```python
from build123d import *

# Parameters (mm, degrees)
SKETCH1_R           = 2.35
BOSS_EXTRUDE1_DEPTH = 7.8
SKETCH2_R           = 2.7
CUT_EXTRUDE1_DEPTH  = 0.7
SKETCH3_R           = 2.705
CUT_EXTRUDE2_DEPTH  = 0.7


with BuildPart() as part:
    # Sketch1 → Boss-Extrude1 (new body)
    with BuildSketch(Plane(origin=(0, 0, 0), x_dir=(0, 0, -1), z_dir=(1, 0, 0))):
        with BuildLine():
            Line((-48, -3.73), (48, -3.73))
            ThreePointArc((48, -3.73), (51.73, 0), (48, 3.73))
            Line((48, 3.73), (-48, 3.73))
            ThreePointArc((-48, 3.73), (-51.73, 0), (-48, -3.73))
        make_face()
        with Locations((-48, 0)):
            Circle(SKETCH1_R, mode=Mode.SUBTRACT)
        with Locations((-40, 0)):
            Circle(SKETCH1_R, mode=Mode.SUBTRACT)
        with Locations((-32, 0)):
            Circle(SKETCH1_R, mode=Mode.SUBTRACT)
        with Locations((-24, 0)):
            Circle(SKETCH1_R, mode=Mode.SUBTRACT)
        with Locations((-16, 0)):
            Circle(SKETCH1_R, mode=Mode.SUBTRACT)
        with Locations((-8, 0)):
            Circle(SKETCH1_R, mode=Mode.SUBTRACT)
        Circle(SKETCH1_R, mode=Mode.SUBTRACT)
        with Locations((8, 0)):
            Circle(SKETCH1_R, mode=Mode.SUBTRACT)
        with Locations((16, 0)):
            Circle(SKETCH1_R, mode=Mode.SUBTRACT)
        with Locations((24, 0)):
            Circle(SKETCH1_R, mode=Mode.SUBTRACT)
        with Locations((32, 0)):
            Circle(SKETCH1_R, mode=Mode.SUBTRACT)
        with Locations((40, 0)):
            Circle(SKETCH1_R, mode=Mode.SUBTRACT)
        with Locations((48, 0)):
            Circle(SKETCH1_R, mode=Mode.SUBTRACT)
    extrude(amount=BOSS_EXTRUDE1_DEPTH)

    # Sketch2 → Cut-Extrude1 (cut)
    with BuildSketch(Plane(origin=(7.8, 0, 0), x_dir=(0, 0, -1), z_dir=(1, 0, 0))):
        with Locations((-48, 0)):
            Circle(SKETCH2_R)
        with Locations((-40, 0)):
            Circle(SKETCH2_R)
        with Locations((-32, 0)):
            Circle(SKETCH2_R)
        with Locations((-24, 0)):
            Circle(SKETCH2_R)
        with Locations((-16, 0)):
            Circle(SKETCH2_R)
        with Locations((-8, 0)):
            Circle(SKETCH2_R)
        Circle(SKETCH2_R)
        with Locations((8, 0)):
            Circle(SKETCH2_R)
        with Locations((16, 0)):
            Circle(SKETCH2_R)
        with Locations((24, 0)):
            Circle(SKETCH2_R)
        with Locations((32, 0)):
            Circle(SKETCH2_R)
        with Locations((40, 0)):
            Circle(SKETCH2_R)
        with Locations((48, 0)):
            Circle(SKETCH2_R)
    extrude(amount=-CUT_EXTRUDE1_DEPTH, mode=Mode.SUBTRACT)

    # Sketch3 → Cut-Extrude2 (cut)
    with BuildSketch(Plane.ZY):
        with Locations((-48, 0)):
            Circle(SKETCH3_R)
        with Locations((-40, 0)):
            Circle(SKETCH3_R)
        with Locations((-32, 0)):
            Circle(SKETCH3_R)
        with Locations((-24, 0)):
            Circle(SKETCH3_R)
        with Locations((-16, 0)):
            Circle(SKETCH3_R)
        with Locations((-8, 0)):
            Circle(SKETCH3_R)
        Circle(SKETCH3_R)
        with Locations((8, 0)):
            Circle(SKETCH3_R)
        with Locations((16, 0)):
            Circle(SKETCH3_R)
        with Locations((24, 0)):
            Circle(SKETCH3_R)
        with Locations((32, 0)):
            Circle(SKETCH3_R)
        with Locations((40, 0)):
            Circle(SKETCH3_R)
        with Locations((48, 0)):
            Circle(SKETCH3_R)
    extrude(amount=-CUT_EXTRUDE2_DEPTH, mode=Mode.SUBTRACT)


solid = part.part
```
Part model, mm, in its own coordinate system. A direction names the side the tool comes from. Coordinates: 2 decimals unless noted, no trailing zeros. Order: outer loops, then holes, each group sorted by start corner. A loop starts at its lowest first (then second) coordinate and runs counter-clockwise, first axis right, second up. Notation, with made-up numbers: (69, -31.75) - (99, -31.75) arc R25 ccw to (99, -13.75) - close; hole circle Ø4 at (-17.5, 2.5). An arc over 180 degrees is marked (long way). Return JSON: item names as keys, results as strings. Group by question number.
Item 1: Pin check, flat tips, straight feed: pin 1 (1 mm diameter, centred on y = 0.5, z = -14.5, fed in from +X); pin 2 (2.5 mm diameter, centred on y = 1, z = -7, fed in from +X); pin 3 (1 mm diameter, centred on x = 5, y = 1.5, fed in from -Z); pin 4 (1.5 mm diameter, centred on x = 3, y = -1.5, fed in from -Z). Stop position of each tip, or through.
Item 2: Pull direction Y, two halves, no side cores. Call faces 1 (the face through (3.855, -2.294, 0.509)), 2 (the face through (0.345, 0.119, -42.702)), 3 (the face through (3.85, -0.08, -51.73)): pulls with the +Y half, pulls with the -Y half, needs draft (parallel to the pull), parting line crosses it, or undercut.
Item 3: Which spindle directions (+Z, -Z, +X, -X, +Y, -Y) get a long thin tool onto all of the face, cutting with end or side? Do faces 4 (the face through (0.35, -2.4, 17.25)), 5 (the face through (7.455, 0.811, -26.575)), 6 (the face through (3.86, -0.9, -10.17)). Say none if no direction does.
Item 4: Cut at A-A (z = -16). List the corners of the cut face in (x, y) (3 decimals).
Item 5: Cut at B-B (x = 4.75). State how many separate pieces and enclosed holes the cut face has, plus the area to 3 significant figures.
Item 6: Drill centre lines: probe 1 along Y at (x, z) = (0.55, 48) (3 decimals); probe 2 along Y at (x, z) = (5.75, -32); probe 3 along X at (y, z) = (-0.75, -42.5). Where is each one in solid material? Low to high. Write a range as from..to.
Check values:
{
 "1": {"pin 1": "passes through", "pin 2": "stops at x = 7.1", "pin 3": "stops at z = -51.59", "pin 4": "stops at z = -51.65"},
 "2": {"face 1": "undercut", "face 2": "undercut", "face 3": "parting line crosses it"},
 "3": {"face 4": "-X", "face 5": "+X", "face 6": "+X, -X"},
 "4": {"outline": "(0, -3.73) - (7.8, -3.73) - (7.8, -2.7) - (7.1, -2.7) - (7.1, -2.35) - (0.7, -2.35) - (0.7, -2.705) - (0, -2.705) - close; (0, 2.705) - (0.7, 2.705) - (0.7, 2.35) - (7.1, 2.35) - (7.1, 2.7) - (7.8, 2.7) - (7.8, 3.73) - (0, 3.73) - close"},
 "5": {"separate pieces": "1", "enclosed holes": "13", "area": "534 mm2"},
 "6": {"probe 1": "y = -3.73..-2.705, 2.705..3.73", "probe 2": "y = -3.73..-2.35, 2.35..3.73", "probe 3": "x = 0.7..7.1"}
}
